CAD build for the part. Positions are in the model's coordinates, mm. Give positions to 0.01 mm unless a question says otherwise; leave off trailing zeros. Order: outer loops, then holes, each group sorted by start corner. A loop starts at its lowest first (then second) coordinate and runs counter-clockwise, first axis right, second up. Notation, with made-up numbers: (60, -38) -> (78, -38) arc R32 ccw to (78, -7) -> close; hole circle Ø9 at (75, 56.5). An arc over 180 degrees is marked (long way). Use one line per item in the form item = value. Start each with the question number.
1) Drop flat-ended pins along their axis: P1, Ø4, axis at x = -7, z = 8, coming from the -Y side; P2, Ø3, axis at y = -37, z = 3.5, coming from the -X side; P3, Ø1.5, axis at y = -3.5, z = 4.5, coming from the +X side. Give the stop position or say it passes through.
2) Cut at A-A, the plane x = 0. Give the cut face in (y, z).
3) Cut at C-C, the plane x = -12. Give the cut face in (y, z), and give its area (3 significant figures).
4) Cut at D-D, the plane z = 4.5. State how many separate pieces and enclosed holes the cut face has, and give its area (3 significant figures).
5) Cut at B-B, the plane y = 21.5. Give the cut face in (x, z).
6) Mould opens along Y. For faces 1 (the face through (-1.08, 4.88, 4.93)), 2 (the face through (-11.875, -18.66, 5.07)), 3 (the face through (-12.657, 18.139, 5.07)), 4 (the face through (54.992, 0.909, 4.93)) say: pulls with the +Y half, pulls with the -Y half, needs draft (parallel to the pull), parting line crosses it, or undercut.
7) Probe line 1 (X direction, y = 0.5, z = 3); line 2 (Y direction, x = -45, z = 6.25); line 3 (X direction, y = 3, z = 3.5). List the from-to ranges inside material, lowest first.
Autodesk Inventor part; units mm, degrees
ref_plane "YZ Plane" through (0, 0, 0) normal (1, 0, 0) x (0, 1, 0)
ref_plane "XZ Plane" through (0, 0, 0) normal (0, 1, 0) x (-1, 0, 0)
ref_plane "XY Plane" through (0, 0, 0) normal (0, 0, 1) x (1, 0, 0)
sketch "Эскиз1" plane through (0, 0, 0) normal (0, 0, 1) x (1, 0, 0)
  circle A0 centre (0, 0) radius 5
  circle A1 centre (0, 0) radius 55
  dimension "d0" = 10
  dimension "d1" = 110
extrude "Выдавливание1" add sketch "Эскиз1" along normal blind 10
sketch "Эскиз2" plane through (0, 0, 10) normal (0, 0, 1) x (1, 0, 0)
  circle A0 centre (-40, 60) radius 50
  line L0 (0, -92.4934) -> (0, 92.4934)
  line L1 (-90.2801, 0) -> (79.2133, 0)
  circle A1 centre (-40, -60) radius 50
  point P0 (0, 0)
  dimension "d4" = 60
  dimension "d5" = 40
  dimension "d14" = 100
extrude "Выдавливание2" cut sketch "Эскиз2" against normal through all
fillet "Сопряжение1" radius 10 4 edges at (9.6561, 54.1457, 5) (-53.6946, 11.912, 5) (9.6561, -54.1457, 5) (-53.6946, -11.912, 5)
fillet_without_effect "Сопряжение2"
sketch "Эскиз3" plane through (0, 0, 10) normal (0, 0, 1) x (1, 0, 0)
  circle A0 centre (0, 0) radius 5
  line L0 (-77, 0) -> (77, 0)
  circle A1 centre (-45, 0) radius 5
  dimension "d10" = 10
  dimension "d11" = 45
extrude "Выдавливание3" cut sketch "Эскиз3" against normal through all contours A1 L0 | L0 A1
properties part number "кривошип_v3"
Result:
q1.P1 = -24.29
q1.P2 = 3.59
q1.P3 = 54.93
q2.outline = (-30, 0) -> (-5, 0) -> (-5, 10) -> (-30, 10) -> close; (5, 0) -> (30, 0) -> (30, 10) -> (5, 10) -> close
q3.outline = (-18.58, 0) -> (18.58, 0) -> (18.58, 10) -> (-18.58, 10) -> close
q3.area = 372 mm²
q4.separate_pieces = 1
q4.enclosed_holes = 2
q4.area = 5,780 mm²
q5.outline = (-8.1, 0) -> (50.62, 0) -> (50.62, 10) -> (-8.1, 10) -> close
q6.face_1 = undercut
q6.face_2 = pulls with the -Y half
q6.face_3 = pulls with the +Y half
q6.face_4 = parting line crosses it
q7.line_1 = -55 to -49.97, -40.03 to -4.97, 4.97 to 55
q7.line_2 = -10.21 to -5, 5 to 10.21
q7.line_3 = -54.6 to -49, -41 to -4, 4 to 54.92
